Could you check a few things on this drawing? It's one solid part, dimensions in mm from its lowest x, y, z. Coordinates: 2 decimals unless noted, no trailing zeros. Order: outer loops, then holes, each group sorted by start corner. A loop starts at its lowest first (then second) coordinate and runs counter-clockwise, first axis right, second up. Notation, with made-up numbers: M 36.25,30 L 62.25,30 A29 cw 62.25,53 Z; hole C -15.75,70 d6. An arc over 180 degrees is marked long. One line per question, with ' | ' between items. Start each with the question number.
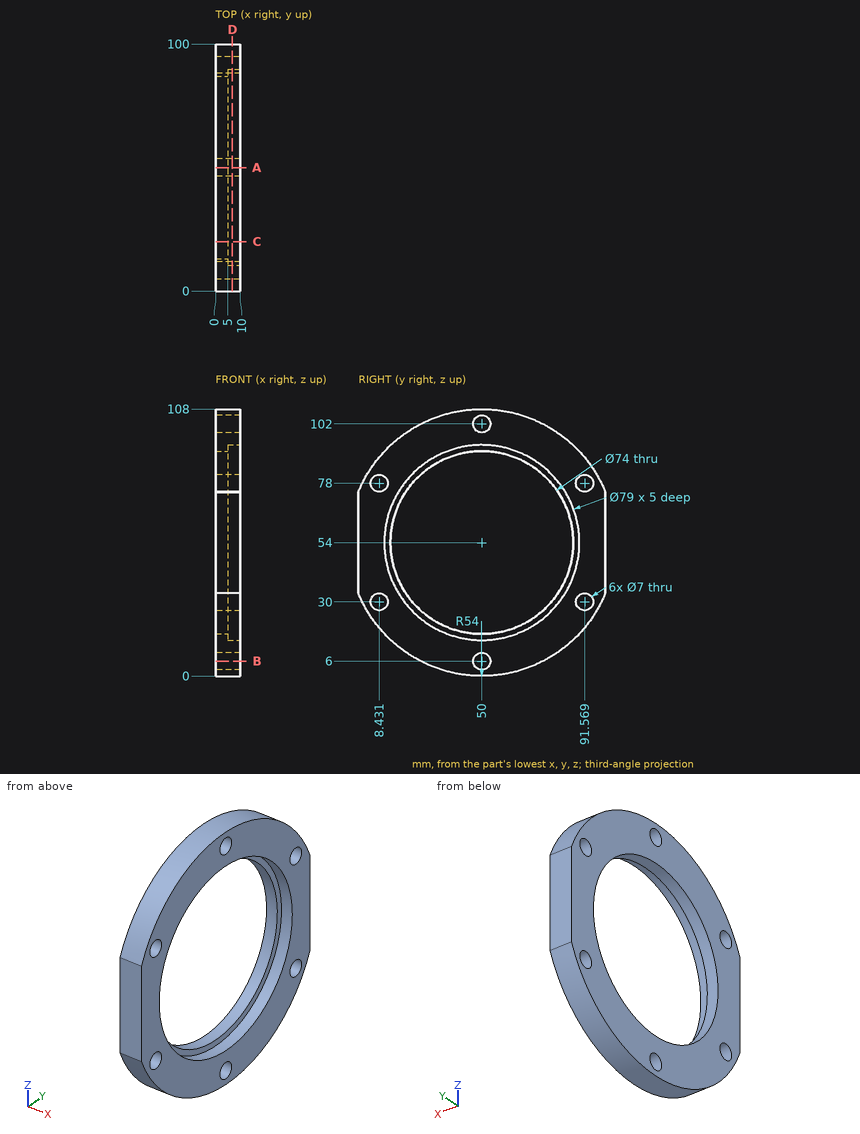
1. Imagine slicing it at B-B (z = 6). List the corners of the cut face in (x, y) for me, then the cut area to 3 significant figures.
2. Will these pins go through, and if not, where does the flat tip stop? pin 1 (6.5 mm diameter, centred on y = 50, z = 102, fed in from -X); pin 2 (4 mm diameter, centred on x = 4, y = 74, fed in from +Z) (1 decimal); pin 3 (9 mm diameter, centred on y = 50, z = 6, fed in from +X); pin 4 (4 mm diameter, centred on x = 9, z = 84, fed in from -Y).
3. Imagine slicing it at C-C (y = 20). List the corners of the cut face in (x, z) for me (1 decimal).
4. Imagine slicing it at D-D (x = 6.75). List the corners of the cut face in (y, z) for me.
5. Imagine slicing it at A-A (y = 50). List the corners of the cut face in (x, z) for me.
6. I need wall thicknesses on line 1 (Z direction, x = 3.75, y = 50); line 2 (Z direction, x = 7.2, y = 50); line 3 (Y direction, x = 3.35, z = 54). Which ranges of each line are inside material? Lowest first, please.
Entries:
1) outline: M 0,25.26 L 10,25.26 L 10,46.5 L 0,46.5 Z; M 0,53.5 L 10,53.5 L 10,74.74 L 0,74.74 Z | area: 425 mm²
2) pin 1: through | pin 2: z = 103.3 | pin 3: x = 10 | pin 4: y = 3.83
3) outline: M 0,9.1 L 10,9.1 L 10,28.3 L 5,28.3 L 5,32.3 L 0,32.3 Z; M 0,75.7 L 5,75.7 L 5,79.7 L 10,79.7 L 10,98.9 L 0,98.9 Z
4) outline: M 0,33.6 A54 ccw 100,33.6 L 100,74.4 A54 ccw 0,74.4 Z; hole C 8.43,30 d7; hole C 8.43,78 d7; hole C 50,54 d79; hole C 50,6 d7; hole C 50,102 d7; hole C 91.57,30 d7; hole C 91.57,78 d7
5) outline: M 0,0 L 10,0 L 10,2.5 L 0,2.5 Z; M 0,9.5 L 10,9.5 L 10,14.5 L 5,14.5 L 5,17 L 0,17 Z; M 0,91 L 5,91 L 5,93.5 L 10,93.5 L 10,98.5 L 0,98.5 Z; M 0,105.5 L 10,105.5 L 10,108 L 0,108 Z
6) line 1: 0 to 2.5, 9.5 to 17, 91 to 98.5, 105.5 to 108 | line 2: 0 to 2.5, 9.5 to 14.5, 93.5 to 98.5, 105.5 to 108 | line 3: 0 to 13, 87 to 100
